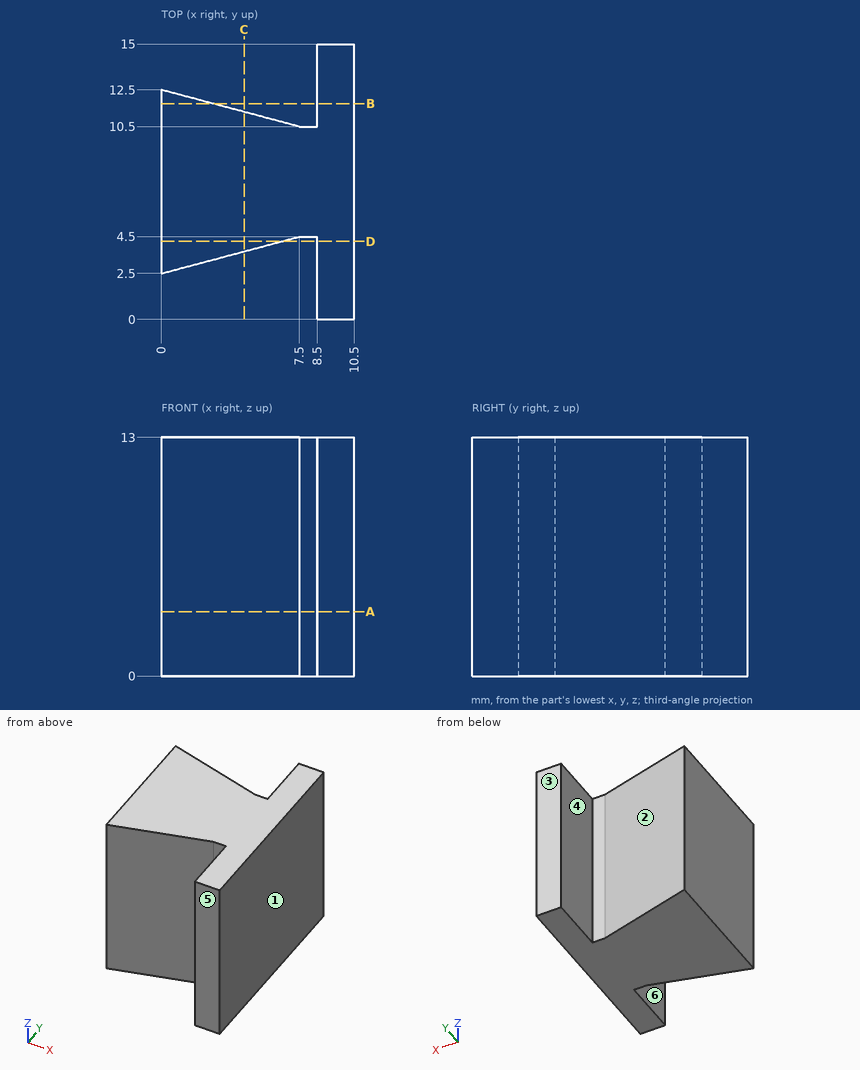
Answer from the drawing. Dimensions are ordinates in mm from the lowest x, y and z of the part. A direction names the side the tool comes from. Give positions to 0.01 mm unless a question says otherwise; leave off trailing zeros. Order: outer loops, then holes, each group sorted by start corner. A loop starts at its lowest first (then second) coordinate and runs counter-clockwise, first axis right, second up.
(1) Find section A-A (z = 3.5). Give the vertices of the cut face in (x, y).
(2) Find section D-D (y = 4.25). Give the vertices of the cut face in (x, z), plus the area to 3 significant figures.
(3) Given pin 1 (0.8 mm diameter, centred on x = 8, z = 7, fed in from -Y); pin 2 (2 mm diameter, centred on x = 4.5, z = 9.5, fed in from -Y); pin 3 (0.5 mm diameter, centred on x = 8, z = 6.5, fed in from +Y), each flat-ended and moving along its own axis, determine where each tip first touches the part or whether it passes through.
(4) For the marked faces 4, 5 and 6, determine the directions among +Z, -Z, +X, -X, +Y, -Y from which every point of the face is accessible in a straight line to the end or side of a thin tool.
(5) For a pull along X with two mould halves and no side action, classify the marked faces 1, 2 and 3 as released by +X, released by -X, zero draft, split by the parting line, or undercut.
(6) Straight lines are drawn through the part: L1, parallel to X at y = 12.75, z = 12; L2, parallel to Y at x = 8.25, z = 1.75; L3, parallel to Y at x = 6.5, z = 10.5. For each, find the intervals that lie inside material, in ascending order.
(7) Find section C-C (x = 4.5). Give the vertices of the cut face in (y, z), plus the area to 3 significant figures.
(8) Find section B-B (y = 11.75). Give the vertices of the cut face in (x, z), plus the area to 3 significant figures.
Result sheet:
1. outline: (0, 2.5) - (7.5, 4.5) - (8.5, 4.5) - (8.5, 0) - (10.5, 0) - (10.5, 15) - (8.5, 15) - (8.5, 10.5) - (7.5, 10.5) - (0, 12.5) - close
2. outline: (0, 0) - (6.56, 0) - (6.56, 13) - (0, 13) - close; (8.5, 0) - (10.5, 0) - (10.5, 13) - (8.5, 13) - close
2. area: 111 mm2
3. pin 1: stops at y = 4.5
3. pin 2: stops at y = 3.43
3. pin 3: stops at y = 10.5
4. face 4: +Z, -Z, +Y
4. face 5: +Z, -Z, +X, -X, -Y
4. face 6: +Z, -Z, -Y
5. face 1: released by +X
5. face 2: undercut
5. face 3: zero draft
6. L1: x = 8.5 to 10.5
6. L2: y = 4.5 to 10.5
6. L3: y = 4.23 to 10.77
7. outline: (3.7, 0) - (11.3, 0) - (11.3, 13) - (3.7, 13) - close
7. area: 98.8 mm2
8. outline: (0, 0) - (2.81, 0) - (2.81, 13) - (0, 13) - close; (8.5, 0) - (10.5, 0) - (10.5, 13) - (8.5, 13) - close
8. area: 62.6 mm2
